Could you check a few things on this model? Use its own coordinates, in mm. Give positions to 0.01 mm unless a question says otherwise; leave off trailing zeros. Loops run counter-clockwise (first coordinate to the right, second up) from the corner with the lowest first, then second, coordinate; pieces in that order, holes last. Notation, with made-up numbers: M 18,-3 L 69,-3 A18 cw 69,4 Z; hole C 3.25,-32.75 d3. An arc over 180 degrees is marked long. Use a Markdown table: item, result. Add a question column.
1) If I drill on line 1 along X through (y, z) = (17, 4.5) (3 decimals); line 2 along Y through (x, z) = (-19, 3); line 3 along Y through (x, z) = (-113.5, 4.5), over which ranges is the centre line in solid material (lowest first)? Write a range as [from, to].
2) Suppose I cut it at B-B on z = 2. List the corners of the cut face in (x, y) for me (3 decimals), and give its area (3 significant figures).
3) Suppose I cut it at C-C on y = -31. List the corners of the cut face in (x, z) for me (3 decimals), and give its area (3 significant figures).
4) Suppose I cut it at A-A on y = 18. List the corners of the cut face in (x, z) for me (3 decimals), and give its area (3 significant figures).
5) Suppose I cut it at D-D on x = 157.5. List the corners of the cut face in (y, z) for me, and give its area (3 significant figures).
6) Will this pin go through, and if not, where does the flat tip stop? pin 1 Ø3 at (x, z) = (5.5, 2) entering from +Y.
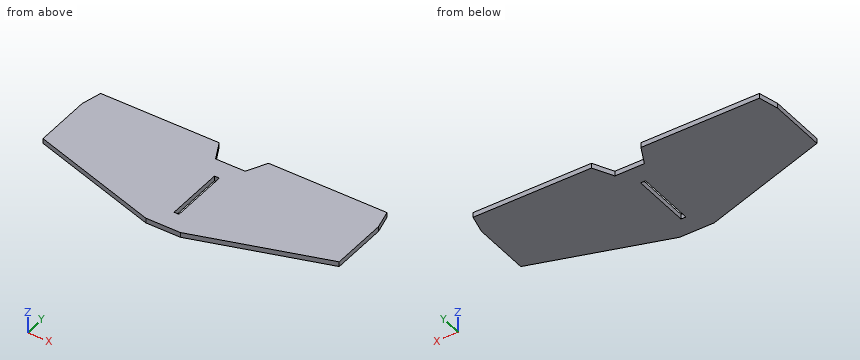
```python
from build123d import *

# Parameters (mm, degrees)
F1_DEPTH = 6.35


with BuildPart() as f1:
    # F0 (on Top) → F1 (new body)
    with BuildSketch(Plane.XY):
        Polygon((-190.5, 63.5), (-190.5, -10.592123), (-22.25318, -63.5), (0, -63.5), (22.25318, -63.5), (190.5, -10.592123), (190.5, 63.5), (19.05, 63.5), (0, 63.5), (-19.05, 63.5), align=None)
        Polygon((3.175, -38.1), (0, -38.1), (-3.175, -38.1), (-3.175, 38.1), (0, 38.1), (3.175, 38.1), align=None, mode=Mode.SUBTRACT)
        Polygon((-184.15, 88.9), (-190.5, 63.5), (-19.05, 63.5), (-31.75, 88.9), align=None)
        Polygon((31.75, 88.9), (19.05, 63.5), (190.5, 63.5), (184.15, 88.9), align=None)
    extrude(amount=F1_DEPTH)


solid = f1.part
```
Answer block:
| question | item | result |
|---|---|---|
| 1 | line 1 | x = [-190.5, -3.175], [3.175, 190.5] |
| 1 | line 2 | y = [-63.5, 63.5] |
| 1 | line 3 | y = [-34.81, 88.9] |
| 2 | outline | M -190.5,-10.592 L -22.253,-63.5 L 22.253,-63.5 L 190.5,-10.592 L 190.5,63.5 L 184.15,88.9 L 31.75,88.9 L 19.05,63.5 L -19.05,63.5 L -31.75,88.9 L -184.15,88.9 L -190.5,63.5 Z; hole M -3.175,-38.1 L 3.175,-38.1 L 3.175,38.1 L -3.175,38.1 Z |
| 2 | area | 47,200 mm^2 |
| 3 | outline | M -125.603,0 L -3.175,0 L -3.175,6.35 L -125.603,6.35 Z; M 3.175,0 L 125.603,0 L 125.603,6.35 L 3.175,6.35 Z |
| 3 | area | 1,550 mm^2 |
| 4 | outline | M -190.5,0 L -3.175,0 L -3.175,6.35 L -190.5,6.35 Z; M 3.175,0 L 190.5,0 L 190.5,6.35 L 3.175,6.35 Z |
| 4 | area | 2,380 mm^2 |
| 5 | outline | M -20.97,0 L 88.9,0 L 88.9,6.35 L -20.97,6.35 Z |
| 5 | area | 698 mm^2 |
| 6 | pin 1 | stops at y = 63.5 |
